Autodesk Inventor part; units mm, degrees
ref_plane "YZ Plane" through (0, 0, 0) normal (1, 0, 0) x (0, 1, 0)
ref_plane "XZ Plane" through (0, 0, 0) normal (0, 1, 0) x (-1, 0, 0)
ref_plane "XY Plane" through (0, 0, 0) normal (0, 0, 1) x (1, 0, 0)
sketch "Sketch1" plane through (0, 0, 0) normal (0, 1, 0) x (-1, 0, 0)
  circle A0 centre (0, 0) radius 5.08
  line L0 (0, 0) -> (0, 3.175)
  line L1 (0, 0) -> (0, -3.175)
  circle A1 centre (0, 0) radius 6.35
  line L2 (0, 3.175) -> (6.35, 0)
  line L3 (0, -3.175) -> (6.35, 0)
  point P0 (5.037429, -0.656286)
  point P1 (5.037429, 0.656286)
  dimension "d3" = 12.7
  dimension "d0" = 10.16
  dimension "d1" = 3.175
  dimension "d2" = 3.175
  dimension "d4" = 6.35
sketch "Sketch1 outline for Extrusion1" plane through (0, 0, 0) normal (0, 1, 0) x (-1, 0, 0)
  line L0 (5.037429, -0.656286) -> (6.35, 0)
  arc A0 (5.037429, 0.656286) -> (5.037429, -0.656286) centre (0, 0) ccw
  line L1 (6.35, 0) -> (5.037429, 0.656286)
extrude "Extrusion1" add sketch "Sketch1 outline for Extrusion1" along normal blind 2.54 draft -10
sketch "Sketch2" plane through (0, 0, 0) normal (0, -1, 0) x (1, 0, 0)
  circle A0 centre (0, 0) radius 1.27
  dimension "d7" = 2.54
extrude "Extrusion2" cut sketch "Sketch2" against normal blind 1.27
properties part number "ChairDial(H)"
The model under review builds one solid part; all positions refer to its coordinate system, in mm. Round coordinates to 2 decimals unless told otherwise and drop trailing zeros. Loops run counter-clockwise (first coordinate to the right, second up) from the corner with the lowest first, then second, coordinate; pieces in that order, holes last. Notation, with made-up numbers: (19.25, -19) -> (41.25, -19) arc R13 cw to (41.25, -8) -> close; hole circle Ø3 at (-22.75, -28.75). An arc over 180 degrees is marked (long way). Answer as a JSON object with one key per item and string values. Group by question number.
1) We need section A-A on x = 0. Write out the cut boundary in (y, z).
2) For line 1 (Z direction, x = 0, y = 0.4); line 2 (Z direction, x = 0.5, y = 0.7); line 3 (Y direction, x = -1, z = 0), list the stretches that pass through material, from the lowest coordinate up. Write a range as [from, to].
3) We need section B-B on y = 1.1. Write out the cut boundary in (x, z).
4) We need section C-C on y = 1.9. Write out the cut boundary in (x, z).
5) We need section D-D on x = -5.5. Write out the cut boundary in (y, z) (3 decimals), then the cut area to 3 significant figures.
6) Mouldability with a two-part tool opening along X and no side actions: class faces 1 (the face through (-5.3, 1.25, -0.28)), 2 (the face through (-0.17, 0.63, 1.26)), 3 (the face through (0, 1.27, 0)), 4 (the face through (4.706, 2.099, -0.202)) as released by +X, released by -X, zero draft, split by the parting line, or undercut.
7) For pin 1 Ø1.5 at (x, y) = (2, 1.5) entering from -Z; pin 2 Ø2 at (x, z) = (0.5, 0) entering from -Y, all flat-tipped, find the tip position at first contact; note any pin that passes through.
Result set:
{
 "1": {"outline": "(0, -5.08) -> (2.54, -4.63) -> (2.54, 4.63) -> (0, 5.08) -> (0, 1.27) -> (1.27, 1.27) -> (1.27, -1.27) -> (0, -1.27) -> close"},
 "2": {"line 1": "[-5.01, -1.27], [1.27, 5.01]", "line 2": "[-4.93, -1.17], [1.17, 4.93]", "line 3": "[1.27, 2.54]"},
 "3": {"outline": "(-5.92, 0) -> (-4.86, -0.53) arc R4.89 ccw (long way) to (-4.86, 0.53) -> close; hole circle Ø2.54 at (0, 0)"},
 "4": {"outline": "(-5.6, 0) -> (-4.72, -0.44) arc R4.74 ccw (long way) to (-4.72, 0.44) -> close"},
 "5": {"outline": "(0, -0.425) -> (2.156, 0) -> (0, 0.425) -> close", "area": "0.916 mm²"},
 "6": {"face 1": "released by -X", "face 2": "undercut", "face 3": "undercut", "face 4": "split by the parting line"},
 "7": {"pin 1": "z = -4.69", "pin 2": "y = 0"}
}
